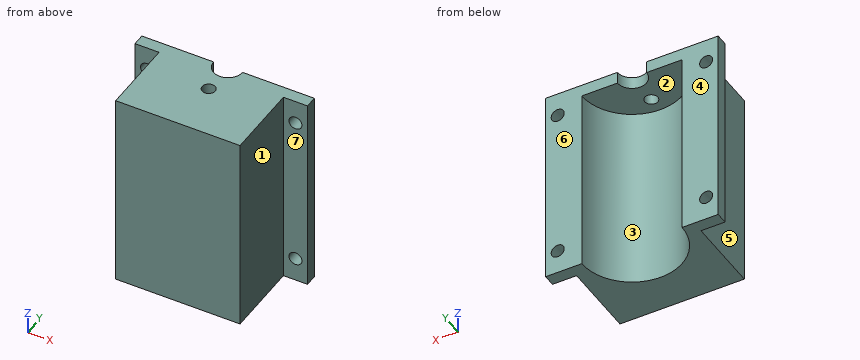
```python
from build123d import *

# Parameters (mm, degrees)
BOSS_EXTRU_1_DEPTH      = 50
ESQUISSE4_R             = 1.625
ENL_V_MAT_EXTRU_1_DEPTH = 50
ESQUISSE7_R             = 1.625
BOSS_EXTRU_2_DEPTH      = 3


with BuildPart() as part:
    # Esquisse1 → Boss.-Extru.1 (new body)
    with BuildSketch(Plane.XY):
        with BuildLine():
            Line((-6, 19), (-6, 22))
            Line((-6, 22), (3, 22))
            ThreePointArc((3, 22), (15.5, 9.5), (28, 22))
            Line((28, 22), (37, 22))
            Line((37, 22), (37, 19))
            Line((37, 19), (31, 19))
            Line((31, 19), (31, 0))
            Line((31, 0), (0, 0))
            Line((0, 0), (0, 19))
            Line((0, 19), (-6, 19))
        make_face()
    extrude(amount=BOSS_EXTRU_1_DEPTH)

    # Esquisse4 → Enlèv. mat.-Extru.1 (cut)
    with BuildSketch(Plane(origin=(0, 22, 0), x_dir=(1, 0, 0), z_dir=(0, 1, 0))):
        with Locations(Location((-3, -44, 0), (0, 0, 270))):
            Circle(ESQUISSE4_R)
        with Locations(Location((34, -44, 0), (0, 0, 270))):
            Circle(ESQUISSE4_R)
        with Locations(Location((34, -6, 0), (0, 0, 270))):
            Circle(ESQUISSE4_R)
        with Locations(Location((-3, -6, 0), (0, 0, 270))):
            Circle(ESQUISSE4_R)
    extrude(amount=-ENL_V_MAT_EXTRU_1_DEPTH, mode=Mode.SUBTRACT)

    # Esquisse7 → Boss.-Extru.2 (add)
    with BuildSketch(Plane.XY.offset(50)):
        with BuildLine():
            Line((19.125, 22), (28, 22))
            Line((28, 22), (28, 9.5))
            Line((28, 9.5), (3, 9.5))
            Line((3, 9.5), (3, 22))
            Line((3, 22), (11.875, 22))
            ThreePointArc((11.875, 22), (15.5, 18.375), (19.125, 22))
        make_face()
        with Locations((15.5, 13.5)):
            Circle(ESQUISSE7_R, mode=Mode.SUBTRACT)
    extrude(amount=-BOSS_EXTRU_2_DEPTH)


solid = part.part
```
Geometry check sheet. Reference: the model listing, model coordinates, mm. Face numbers are marked on the shaded views. A direction names the side the tool comes from. Give positions to 0.01 mm unless a question says otherwise; leave off trailing zeros. Loops run counter-clockwise (first coordinate to the right, second up) from the corner with the lowest first, then second, coordinate; pieces in that order, holes last. Notation, with made-up numbers: M 73.25,89.5 L 125.25,89.5 A15 ccw 125.25,96.5 Z; hole C -22.5,-16.75 d11. An arc over 180 degrees is marked long. Write item = value, one per line.
(1) Tool access check on the marked faces 5, 6 and 7. Record the directions out of +Z, -Z, +X, -X, +Y, -Y that give a thin tool (end or side, any length) a straight path to the whole face; none if there is none.
Answer below:
face_5 = +Z, -Z, -X, -Y
face_6 = +Z, -Z, +X, -X, +Y
face_7 = +Z, -Z, +X, -Y
(2) Sectioned sample at B-B, the plane y = 20.25. Record the cut outline in (x, z) (3 decimals), plus the area to 3 significant figures.
Answer below:
outline = M -6,0 L 3.123,0 L 3.123,47 L 12.325,47 L 12.325,50 L -6,50 Z; M 18.675,47 L 27.877,47 L 27.877,0 L 37,0 L 37,50 L 18.675,50 Z; hole C -3,6 d3.25; hole C -3,44 d3.25; hole C 34,6 d3.25; hole C 34,44 d3.25
area = 934 mm2
(3) Sectioned sample at C-C, the plane z = 44. Record the cut outline in (x, y) (3 decimals).
Answer below:
outline = M -6,19 L -4.625,19 L -4.625,22 L -6,22 Z; M -1.375,19 L 0,19 L 0,0 L 31,0 L 31,19 L 32.375,19 L 32.375,22 L 28,22 A12.5 cw 3,22 L -1.375,22 Z; M 35.625,19 L 37,19 L 37,22 L 35.625,22 Z
(4) Release check for a two-part mould opening along X. For the marked faces 1, 2, 3 and 4 record: released by +X, released by -X, zero draft, split by the parting line, or undercut.
Answer below:
face_1 = released by +X
face_2 = undercut
face_3 = undercut
face_4 = zero draft
(5) Gauge pin test, flat ends, axial feed: pin 1 Ø10 at (y, z) = (3.5, 20.5) entering from +X; pin 2 Ø1 at (x, z) = (32.5, 44) entering from -Y; pin 3 Ø8 at (x, z) = (10, 37) entering from +Y. Record the tip position at first contact, or that the pin passes through.
Answer below:
pin_1 = 31
pin_2 = 19
pin_3 = 13.88
(6) Material ranges on line 1 (X direction, y = 19.9, z = 6) (3 decimals); line 2 (Y direction, x = -1.5, z = 21); line 3 (Y direction, x = 15.5, z = 48.75) (3 decimals), recorded low to high. Write a range as [from, to].
Answer below:
line_1 = [-6, -4.625], [-1.375, 3.178], [27.822, 32.375], [35.625, 37]
line_2 = [19, 22]
line_3 = [0, 11.875], [15.125, 18.375]
(7) Sectioned sample at D-D, the plane x = 34. Record the cut outline in (y, z) (3 decimals).
Answer below:
outline = M 19,0 L 22,0 L 22,4.375 L 19,4.375 Z; M 19,7.625 L 22,7.625 L 22,42.375 L 19,42.375 Z; M 19,45.625 L 22,45.625 L 22,50 L 19,50 Z
(8) Sectioned sample at A-A, the plane x = 15.5. Record the cut outline in (y, z) (3 decimals).
Answer below:
outline = M 0,0 L 9.5,0 L 9.5,47 L 11.875,47 L 11.875,50 L 0,50 Z; M 15.125,47 L 18.375,47 L 18.375,50 L 15.125,50 Z
